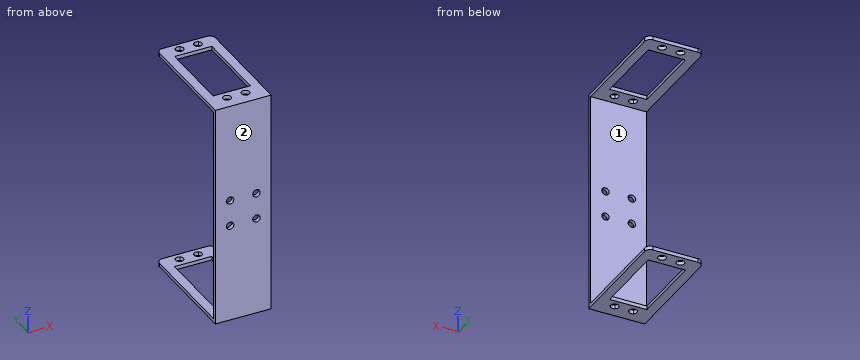
Autodesk Inventor part; units mm, degrees
ref_plane "YZ Plane" through (0, 0, 0) normal (1, 0, 0) x (0, 1, 0)
ref_plane "XZ Plane" through (0, 0, 0) normal (0, 1, 0) x (-1, 0, 0)
ref_plane "XY Plane" through (0, 0, 0) normal (0, 0, 1) x (1, 0, 0)
sketch "Sketch1" plane through (0, 0, 0) normal (0, 1, 0) x (-1, 0, 0)
  line L0 (-15, 60) -> (15, 60)
  line L1 (15, 60) -> (15, -60)
  line L2 (15, -60) -> (-15, -60)
  line L3 (-15, -60) -> (-15, 60)
  line L4 (-15, 60) -> (15, -60) construction
  line L5 (15, 60) -> (-15, -60) construction
  circle A0 centre (7.0711, -7.0711) radius 2
  line L6 (7.0711, -7.0711) -> (0, 0) construction
  circle A1 centre (0, 0) radius 65.2762 construction
  circle A2 centre (7.0711, 7.0711) radius 2
  circle A3 centre (-7.0711, 7.0711) radius 2
  circle A4 centre (-7.0711, -7.0711) radius 2
  dimension "d0" = 30
  dimension "d1" = 120
  dimension "d2" = 10
  dimension "d3" = 4
  dimension "d4" = 45
  dimension "d7" = 360
extrude "Extrusion1" add sketch "Sketch1" along normal blind 2
sketch "Sketch2" plane through (0, 2, 0) normal (0, 1, 0) x (1, 0, 0)
  line L0 (15, 60) -> (-15, 60)
  line L1 (-15, 60) -> (15, 60)
  line L2 (15, 60) -> (15, 58)
  line L3 (15, 58) -> (-15, 58)
  line L4 (-15, 58) -> (-15, 60)
  line L5 (15, -60) -> (15, 60)
  point P0 (0, 0)
  dimension "d11" = 2
extrude "Extrusion2" add sketch "Sketch2" along normal blind 62
sketch "Sketch3" plane through (15, 0, -60) normal (0, 0, -1) x (-1, 0, 0)
  line L0 (5, 55) -> (25, 55)
  line L1 (25, 55) -> (25, 15)
  line L2 (25, 15) -> (5, 15)
  line L3 (5, 15) -> (5, 55)
  line L4 (0, 0) -> (0, 64)
  line L5 (0, 64) -> (30, 64)
  point P0 (15, 0)
  dimension "d14" = 40
  dimension "d15" = 20
  dimension "d16" = 5
  dimension "d17" = 9
extrude "Extrusion3" cut sketch "Sketch3" against normal up to surface (2 mm away)
fillet "Fillet1" radius 3 2 edges at (15, 64, -59) (-15, 64, -59)
mirror "Mirror1" about plane through (0, 0, 0) normal (0, 0, 1) of "Extrusion2", "Extrusion3", "Fillet1"
sketch "Sketch4" plane through (15, 0, -60) normal (0, 0, -1) x (-1, 0, 0)
  arc A0 (21.05, 8.7294) -> (18.64, 8.7294) centre (19.845, 10.51) ccw construction
  arc A1 (11.18, 8.7294) -> (8.77, 8.7294) centre (9.975, 10.51) ccw construction
  line L0 (11.18, 8.25) -> (11.18, 8.7294) construction
  line L1 (11.18, 8.25) -> (18.64, 8.25) construction
  line L2 (18.64, 8.7294) -> (18.64, 8.25) construction
  arc A2 (21.05, 8.7294) -> (18.64, 8.7294) centre (19.845, 10.51) ccw construction
  line L3 (21.05, 8.25) -> (21.05, 8.7294) construction
  line L4 (21.05, 8.25) -> (24.13, 8.25) construction
  line L5 (24.13, 8.25) -> (24.13, 15.0287) construction
  spline S0 degree 2 poles (24.13, 15.0287) (23.9893, 15) (23.82, 15) knots 0.830662 0.830662 0.830662 1 1 1 construction
  line L6 (23.82, 15) -> (6, 15) construction
  spline S1 degree 2 poles (6, 15) (5.8307, 15) (5.69, 15.0287) knots -1 -1 -1 -0.830662 -0.830662 -0.830662 construction
  line L7 (5.69, 8.25) -> (5.69, 15.0287) construction
  line L8 (5.69, 8.25) -> (8.77, 8.25) construction
  line L9 (8.77, 8.7294) -> (8.77, 8.25) construction
  arc A3 (18.64, 61.5906) -> (21.05, 61.5906) centre (19.845, 59.81) ccw
  arc A4 (8.77, 61.5906) -> (11.18, 61.5906) centre (9.975, 59.81) ccw
  circle A5 centre (19.845, 59.81) radius 2.15
  circle A6 centre (9.975, 59.81) radius 2.15
  arc A7 (21.05, 8.7294) -> (18.64, 8.7294) centre (19.845, 10.51) ccw
  arc A8 (11.18, 8.7294) -> (8.77, 8.7294) centre (9.975, 10.51) ccw
  circle A9 centre (19.845, 10.51) radius 2.15
  circle A10 centre (9.975, 10.51) radius 2.15
  point P0 (15, 0)
  point P1 (21.05, 8.7294)
  point P2 (11.18, 8.7294)
  point P3 (21.05, 61.5906)
  point P4 (11.18, 61.5906)
extrude "Extrusion4" cut sketch "Sketch4" against normal through all
sketch "Sketch5" plane through (0, 2, 0) normal (0, 1, 0) x (1, 0, 0)
  line L0 (-15, 60) -> (-15, -60)
  line L1 (-15, -58) -> (15, -58)
  line L2 (15, -58) -> (15, 58)
  line L3 (15, 58) -> (-15, 58)
  line L4 (-15, 58) -> (-15, -58)
  circle A0 centre (-7.0711, 7.0711) radius 2
  circle A1 centre (-7.0711, -7.0711) radius 2
  circle A2 centre (7.0711, -7.0711) radius 2
  circle A3 centre (7.0711, 7.0711) radius 2
  point P0 (0, 0)
  point P1 (-15, 58)
extrude "Extrusion5" add sketch "Sketch5" along normal blind 3
sketch "Sketch6" plane through (0, 0, 0) normal (0, -1, 0) x (1, 0, 0)
  line L0 (15, -60) -> (-15, -60)
  line L1 (15, 60) -> (15, -60)
  line L2 (-15, 60) -> (15, 60)
  line L3 (-15, -60) -> (-15, 60)
  circle A0 centre (7.0711, -7.0711) radius 2
  circle A1 centre (7.0711, 7.0711) radius 2
  circle A2 centre (-7.0711, 7.0711) radius 2
  circle A3 centre (-7.0711, -7.0711) radius 2
  point P0 (0, 0)
extrude "Extrusion6" cut sketch "Sketch6" against normal blind 3
properties part number "new-motor-base"
Model file for the job. Use its own axes, mm. Face numbers are marked on the shaded views. Round coordinates to 2 decimals unless told otherwise and drop trailing zeros. Loops run counter-clockwise (first coordinate to the right, second up) from the corner with the lowest first, then second, coordinate; pieces in that order, holes last.
1. Band-saw the part on C-C, the plane x = -0.5. List the corners of the cut face in (y, z), and give its area (3 significant figures).
Check values:
outline: (3, -60) - (15, -60) - (15, -58) - (5, -58) - (5, 58) - (15, 58) - (15, 60) - (3, 60) - close; (55, -60) - (64, -60) - (64, -58) - (55, -58) - close; (55, 58) - (64, 58) - (64, 60) - (55, 60) - close
area: 316 mm2
2. Band-saw the part on D-D, the plane z = -30. List the corners of the cut face in (x, y), and give its area (3 significant figures).
Check values:
outline: (-15, 3) - (15, 3) - (15, 5) - (-15, 5) - close
area: 60.0 mm2
3. Band-saw the part on A-A, the plane y = 10.51. List the corners of the cut face in (x, z).
Check values:
outline: (-15, -60) - (-7, -60) - (-7, -58) - (-15, -58) - close; (-15, 58) - (-7, 58) - (-7, 60) - (-15, 60) - close; (-2.69, -60) - (2.87, -60) - (2.87, -58) - (-2.69, -58) - close; (-2.69, 58) - (2.87, 58) - (2.87, 60) - (-2.69, 60) - close; (7.18, -60) - (15, -60) - (15, -58) - (7.18, -58) - close; (7.18, 58) - (15, 58) - (15, 60) - (7.18, 60) - close
4. Mould opens along Z. For the marked faces 1 and 2 say: +Z half, -Z half, draft (parallel to the pull), parting line (faces both ways), or undercut.
Check values:
face 1: undercut
face 2: draft
5. Wall check: probe 1 along X at (y, z) = (59.81, 58.6); probe 2 along Z at (x, y) = (4, 57.5); probe 3 along Y at (x, z) = (-4.75, 34). Give the ranges that are in metal, low to high.
Check values:
probe 1: x = -15 to -7, -2.69 to 2.87, 7.18 to 15
probe 2: z = -60 to -58, 58 to 60
probe 3: y = 3 to 5
6. Band-saw the part on B-B, the plane y = 37.5. List the corners of the cut face in (x, z), and give its area (3 significant figures).
Check values:
outline: (-15, -60) - (-10, -60) - (-10, -58) - (-15, -58) - close; (-15, 58) - (-10, 58) - (-10, 60) - (-15, 60) - close; (10, -60) - (15, -60) - (15, -58) - (10, -58) - close; (10, 58) - (15, 58) - (15, 60) - (10, 60) - close
area: 40.0 mm2
